Geometry check sheet. Reference: the model listing, model coordinates, mm. A direction names the side the tool comes from. Round coordinates to 2 decimals unless told otherwise and drop trailing zeros. Order: outer loops, then holes, each group sorted by start corner. A loop starts at its lowest first (then second) coordinate and runs counter-clockwise, first axis right, second up. Notation, with made-up numbers: (59, 70) -> (114, 70) arc R8 cw to (114, 82) -> close; hole circle Ø1 at (79, -11.75). An arc over 180 degrees is marked (long way). Answer as a JSON object with one key per item and string values. Group by question number.
from build123d import *

# Parameters (mm, degrees)
BOSS_EXTRUDE1_DEPTH = 90
FILLET3_R           = 3.75
BOSS_EXTRUDE2_REACH = 132.814
FILLET4_R           = 5
SKETCH5_R           = 4.75
BOSS_EXTRUDE7_DEPTH = 23
CUT_EXTRUDE2_DEPTH  = 6.8
CUT_EXTRUDE3_REACH  = 125.885
SKETCH7_R           = 1.75
CHAMFER1_SIZE       = 8
FILLET5_R           = 5
CUT_EXTRUDE4_START  = -94
SKETCH8_W           = 125.822690829
SKETCH8_H           = 77.860904062
CUT_EXTRUDE4_DEPTH  = 94
SKETCH9_R           = 10
CUT_EXTRUDE5_DEPTH  = 10
SKETCH10_R          = 5
CUT_EXTRUDE6_DEPTH  = 56


# Read off the part's stored shape, not the designer's step: Mirror1
# Some blends are built 0.0001 mm under size
with BuildPart() as part:
    # Sketch2 → Boss-Extrude1 (new body)
    with BuildSketch(Plane(origin=(0, 0, 0), x_dir=(0, 0, -1), z_dir=(1, 0, 0))):
        Polygon((-1.111261719, 3), (46.888738281, 3), (46.888738281, 6.639528096), (58.388738281, 13.279056191), (69.888738281, 6.639528096), (69.888738281, -6.639528096), (58.388738281, -13.279056191), (46.888738281, -6.639528096), (46.888738281, -3), (-1.111261719, -3), (-1.111261719, -6.639528096), (-12.611261719, -13.279056191), (-24.111261719, -6.639528096), (-24.111261719, 6.639528096), (-12.611261719, 13.279056191), (-1.111261719, 6.639528096), align=None)
    extrude(amount=BOSS_EXTRUDE1_DEPTH)

    # Fillet3
    # the kernel refuses this fillet: 3.75 mm, written as the material it adds along each edge
    with BuildSketch(Plane(origin=(0, -3, 1.111261719), x_dir=(0, 0, -1), z_dir=(1, 0, 0)), Plane(origin=(0, 3, -46.888738281), x_dir=(0, 0, 1), z_dir=(1, 0, 0))) as fillet3_piece_1:
        with BuildLine():
            CenterArc((3.748372441, -3.75), FILLET3_R, 90, 88.311869402)
            Line((0, -3.639528096), (-0.074967449, -3.637318658))
            ThreePointArc((-0.074967449, -3.637318658), (-0.075, -1.819764048), (-0.075, 0))
            Line((-0.075, 0), (0, 0.075))
            Line((0, 0.075), (3.748372441, 0.075))
            Line((3.748372441, 0.075), (3.748372441, 0))
        make_face()
    extrude(amount=90)
    with BuildSketch(Plane(origin=(0, -3, -46.888738281), x_dir=(0, -1, 0), z_dir=(1, 0, 0))) as fillet3_piece_2:
        with BuildLine():
            CenterArc((3.75, -3.748372441), FILLET3_R, 91.688130598, 88.311869402)
            Line((0, -3.748372441), (-0.075, -3.748372441))
            Line((-0.075, -3.748372441), (-0.075, 0))
            Line((-0.075, 0), (0, 0.075))
            ThreePointArc((0, 0.075), (1.819764048, 0.075), (3.637318658, 0.074967449))
            Line((3.637318658, 0.074967449), (3.639528096, 0))
        make_face()
    extrude(amount=90)
    with BuildSketch(Plane(origin=(0, 3, 1.111261719), x_dir=(0, 0, -1), z_dir=(1, 0, 0))) as fillet3_piece_3:
        with BuildLine():
            CenterArc((3.748372441, 3.75), FILLET3_R, 181.688130598, 88.311869402)
            Line((0, 3.639528096), (-0.074967449, 3.637318658))
            ThreePointArc((-0.074967449, 3.637318658), (-0.075, 1.819764048), (-0.075, 0))
            Line((-0.075, 0), (0, -0.075))
            Line((0, -0.075), (3.748372441, -0.075))
            Line((3.748372441, -0.075), (3.748372441, 0))
        make_face()
    extrude(amount=90)

    # Boss-Extrude2: up to this face of the body (flat: up to its plane)
    boss_extrude2_end = Plane(part.part.faces().sort_by_distance((45, 0, 24.111261719))[0])
    # Sketch4 → Boss-Extrude2 (add, up to the picked face)
    with BuildSketch(Plane(origin=(0, 0, -69.888738281), x_dir=(-1, 0, 0), z_dir=(0, 0, -1)), mode=Mode.PRIVATE) as boss_extrude2_sk1:
        with BuildLine():
            Line((-46, 3), (-46, 17.64593212))
            ThreePointArc((-46, 17.64593212), (-52.426589902, 29.964512656), (-43.5, 40.611788219))
            Line((-43.5, 40.611788219), (-43.5, 48.611788219))
            Line((-43.5, 48.611788219), (-40.5, 48.611788219))
            Line((-40.5, 48.611788219), (-40.5, 41.101784216))
            Line((-40.5, 41.101784216), (-40.5, 38.0986212))
            ThreePointArc((-40.5, 38.0986212), (-40, 19.111788219), (-39.5, 38.0986212))
            Line((-39.5, 38.0986212), (-39.5, 41.101784216))
            Line((-39.5, 41.101784216), (-39.5, 48.611788219))
            Line((-39.5, 48.611788219), (-36.5, 48.611788219))
            Line((-36.5, 48.611788219), (-36.5, 40.611788219))
            ThreePointArc((-36.5, 40.611788219), (-27.573410098, 29.964512656), (-34, 17.64593212))
            Line((-34, 17.64593212), (-34, 3))
            Line((-34, 3), (-46, 3))
        make_face()
    boss_extrude2_tool1 = split(extrude(boss_extrude2_sk1.sketch, amount=-BOSS_EXTRUDE2_REACH, mode=Mode.PRIVATE), bisect_by=boss_extrude2_end, keep=Keep.BOTH, mode=Mode.PRIVATE)
    add(boss_extrude2_tool1.solids().sort_by(Axis((45.479862, 10.322966, -69.888738), (0, 0, 1)))[0])

    # Fillet4
    fillet4_edges = [part.edges().sort_by_distance(p)[0] for p in [
        (34, 17.64593212, -22.888738281),
        (46, 17.64593212, -22.888738281),
    ]]
    fillet(fillet4_edges, radius=FILLET4_R)

    # Sketch5 → Boss-Extrude7 (add)
    with BuildSketch(Plane(origin=(0, 0, -69.888738281), x_dir=(-1, 0, 0), z_dir=(0, 0, -1))):
        with BuildLine():
            Line((-84, 28.611788219), (-84, 6.639528096))
            Line((-84, 6.639528096), (-53, 6.639528096))
            Line((-53, 6.639528096), (-53, 28.611788219))
            ThreePointArc((-53, 28.611788219), (-68.5, 44.111788219), (-84, 28.611788219))
        make_face()
        with Locations((-68.5, 28.611788219)):
            Circle(SKETCH5_R, mode=Mode.SUBTRACT)
    extrude(amount=-BOSS_EXTRUDE7_DEPTH)

    # Sketch6 → Cut-Extrude2 (cut)
    with BuildSketch(Plane.XY.offset(-46.888738281)):
        Polygon((60.994446501, 28.611788219), (64.74722325, 22.111788219), (72.25277675, 22.111788219), (76.005553499, 28.611788219), (72.25277675, 35.111788219), (64.74722325, 35.111788219), align=None)
    extrude(amount=-CUT_EXTRUDE2_DEPTH, mode=Mode.SUBTRACT)

    # Cut-Extrude3: up to this face of the body (flat: up to its plane)
    cut_extrude3_end = Plane(part.part.faces().sort_by_distance((53, 19.187065128, -58.388738281))[0])
    # Sketch7 → Cut-Extrude3 (cut, up to the picked face)
    with BuildSketch(Plane.ZY, mode=Mode.PRIVATE) as cut_extrude3_sk1:
        with Locations((10.111261719, 44.611788219)):
            Circle(SKETCH7_R)
    cut_extrude3_tool1 = split(extrude(cut_extrude3_sk1.sketch, amount=-CUT_EXTRUDE3_REACH, mode=Mode.PRIVATE), bisect_by=cut_extrude3_end, keep=Keep.BOTH, mode=Mode.PRIVATE)
    # Sketch7 → Cut-Extrude3 (cut, up to the picked face)
    with BuildSketch(Plane.ZY, mode=Mode.PRIVATE) as cut_extrude3_sk2:
        with Locations((-55.888738281, 44.611788219)):
            Circle(SKETCH7_R)
    cut_extrude3_tool2 = split(extrude(cut_extrude3_sk2.sketch, amount=-CUT_EXTRUDE3_REACH, mode=Mode.PRIVATE), bisect_by=cut_extrude3_end, keep=Keep.BOTH, mode=Mode.PRIVATE)
    # Sketch7 → Cut-Extrude3 (cut, up to the picked face)
    with BuildSketch(Plane.ZY, mode=Mode.PRIVATE) as cut_extrude3_sk3:
        Polygon((-41.888738281, 40.611788219), (-22.888738281, 21.611788219), (-3.888738281, 40.611788219), (-3.888738281, 48.611788219), (-41.888738281, 48.611788219), align=None)
    cut_extrude3_tool3 = split(extrude(cut_extrude3_sk3.sketch, amount=-CUT_EXTRUDE3_REACH, mode=Mode.PRIVATE), bisect_by=cut_extrude3_end, keep=Keep.BOTH, mode=Mode.PRIVATE)
    add(cut_extrude3_tool1.solids().sort_by(Axis((0, 44.611788, 10.111262), (1, 0, 0)))[0], mode=Mode.SUBTRACT)
    add(cut_extrude3_tool2.solids().sort_by(Axis((0, 44.611788, -55.888738), (1, 0, 0)))[0], mode=Mode.SUBTRACT)
    add(cut_extrude3_tool3.solids().sort_by(Axis((0, 39.002264, -22.888738), (1, 0, 0)))[0], mode=Mode.SUBTRACT)

    # Chamfer1
    chamfer1_edges = [part.edges().sort_by_distance(p)[0] for p in [
        (42, 48.611788219, -41.888738281),
        (42, 48.611788219, -69.888738281),
        (42, 48.611788219, -3.888738281),
        (42, 48.611788219, 24.111261719),
        (38, 48.611788219, -41.888738281),
        (38, 48.611788219, -69.888738281),
        (38, 48.611788219, -3.888738281),
        (38, 48.611788219, 24.111261719),
    ]]
    chamfer(chamfer1_edges, length=CHAMFER1_SIZE - 0.0001)  # a hair under: the kernel refuses the full size

    # Fillet5
    fillet5_edges = [part.edges().sort_by_distance(p)[0] for p in [
        (42, 48.611788219, -49.888638281),
        (42, 48.611788219, -61.888838281),
        (38, 48.611788219, -49.888638281),
        (38, 48.611788219, -61.888838281),
        (42, 48.611788219, 16.111361719),
        (42, 48.611788219, 4.111161719),
        (38, 48.611788219, 16.111361719),
        (38, 48.611788219, 4.111161719),
    ]]
    fillet(fillet5_edges, radius=FILLET5_R)

    # Mirror1: part across plane


with BuildPart() as part_1:
    add(part.part)
    add(part.part.mirror(Plane.ZY.offset(-90)))

    # Sketch8 → Cut-Extrude4 (cut)
    with BuildSketch(Plane.XY.offset(24.111261719).offset(CUT_EXTRUDE4_START)):
        with Locations((27.088654585, 25.65139584)):
            Rectangle(SKETCH8_W, SKETCH8_H)
    extrude(amount=CUT_EXTRUDE4_DEPTH, mode=Mode.SUBTRACT)

    # Sketch9 → Cut-Extrude5 (cut)
    with BuildSketch(Plane.XZ.offset(3)):
        with Locations(Location((106, -22.888738281, 0), (0, 0, 270))):
            Circle(SKETCH9_R)
    extrude(amount=-CUT_EXTRUDE5_DEPTH, mode=Mode.SUBTRACT)

    # Sketch10 → Cut-Extrude6 (cut)
    with BuildSketch(Plane.ZY.offset(-90)):
        with Locations((12.611261719, 0)):
            Circle(SKETCH10_R)
        with Locations((-58.388738281, 0)):
            Circle(SKETCH10_R)
    extrude(amount=-CUT_EXTRUDE6_DEPTH, mode=Mode.SUBTRACT)


solid = part_1.part
Item 1: Sectioned sample at A-A, the plane x = 100.5. Enter the section's corners in (y, z).
Item 2: Depth check by flat-ended pin: pin 1 Ø6 at (x, y) = (155, 20.5) entering from -Z; pin 2 Ø10.5 at (x, y) = (109.5, 27.5) entering from +Z; pin 3 Ø3 at (y, z) = (41, 1.5) entering from +X; pin 4 Ø9.5 at (y, z) = (10, -12.5) entering from +X. Enter the tip coordinate at first touch or a pass-through.
Item 3: Thickness scan on L1, parallel to X at y = 45, z = 19; L2, parallel to X at y = 28, z = -9.5; L3, parallel to Y at x = 151, z = -12. Record the ranges inside material, lowest first.
Item 4: Sectioned sample at D-D, the plane y = 31.5. Enter the section's corners in (x, z), then the cut area to 3 significant figures.
Item 5: Sectioned sample at B-B, the plane y = 0. Enter the section's corners in (x, z), then the cut area to 3 significant figures.
Item 6: Mould release check, pull along Z, two halves, no side actions. Record for faces 5 (the flat face through (163.238, 9.913, 18.442)), 6 (the flat face through (143.5, 42, -56)), 7 (the flat face through (142, 43.8, -0.7)): pulls with the +Z half, pulls with the -Z half, needs draft (parallel to the pull), parting line crosses it, or undercut.
Item 7: Set-up check for faces 1 (the cylindrical face through (163.24, 4.03, -45.72)), 2 (the cylindrical face through (117.61, -1.92, -53.77)), 3 (the flat face through (135.63, -10.006, -52.719)), 4 (the flat face through (93.042, 9.913, -52.558)): record each of +Z, -Z, +X, -X, +Y, -Y from which the full face is reachable in a straight line by a thin tool's end or side.
Item 8: Sectioned sample at C-C, the plane x = 111.5. Count the separate pieces of the cut face and the enclosed holes in it, then the cut area to 3 significant figures.
Result:
{
 "1": {"outline": "(-13.28, -58.39) -> (-6.64, -69.89) -> (39.53, -69.89) -> (39.53, -46.89) -> (6.64, -46.89) arc R3.75 cw to (3, -43.14) -> (3, -31.24) -> (-3, -31.24) -> (-3, -43.14) arc R3.75 cw to (-6.64, -46.89) -> close; (-13.28, 12.61) -> (-6.64, 1.11) arc R3.75 cw to (-3, -2.64) -> (-3, -14.54) -> (3, -14.54) -> (3, -2.64) arc R3.75 cw to (6.64, 1.11) -> (13.28, 12.61) -> (6.64, 24.11) -> (-6.64, 24.11) -> close; hole circle Ø10 at (0, -58.39); hole circle Ø10 at (0, 12.61)"},
 "2": {"pin 1": "passes through", "pin 2": "stops at z = -46.89", "pin 3": "stops at x = 146.14", "pin 4": "stops at x = 146"},
 "3": {"L1": "x = 136.5 to 139.5, 140.5 to 143.5", "L2": "x = 127.51 to 130.52, 149.48 to 152.49", "L3": "y = -3 to 3, 22.67 to 32.5"},
 "4": {"outline": "(96.27, -69.89) -> (107.73, -69.89) -> (107.73, -53.69) -> (105.66, -53.69) -> (105.66, -46.89) -> (96.27, -46.89) -> close; (115.27, -69.89) -> (126.73, -69.89) -> (126.73, -46.89) -> (117.34, -46.89) -> (117.34, -53.69) -> (115.27, -53.69) -> close; (127.84, -69.89) -> (130.95, -69.89) -> (130.95, -32.78) -> (127.84, -32.78) -> close; (127.84, -13) -> (130.95, -13) -> (130.95, 24.11) -> (127.84, 24.11) -> close; (149.05, -69.89) -> (152.16, -69.89) -> (152.16, -32.78) -> (149.05, -32.78) -> close; (149.05, -13) -> (152.16, -13) -> (152.16, 24.11) -> (149.05, 24.11) -> close", "area": "961 mm2"},
 "5": {"outline": "(90, -69.89) -> (180, -69.89) -> (180, 24.11) -> (90, 24.11) -> (90, 17.61) -> (146, 17.61) -> (146, 7.61) -> (90, 7.61) -> (90, -53.39) -> (146, -53.39) -> (146, -63.39) -> (90, -63.39) -> close; hole circle Ø20 at (106, -22.89)", "area": "7,030 mm2"},
 "6": {"face 5": "pulls with the +Z half", "face 6": "needs draft", "face 7": "undercut"},
 "7": {"face 1": "+X", "face 2": "-X", "face 3": "+X, -X, -Y", "face 4": "-X, +Y"},
 "8": {"separate pieces": "3", "enclosed holes": "2", "area": "1,500 mm2"}
}
